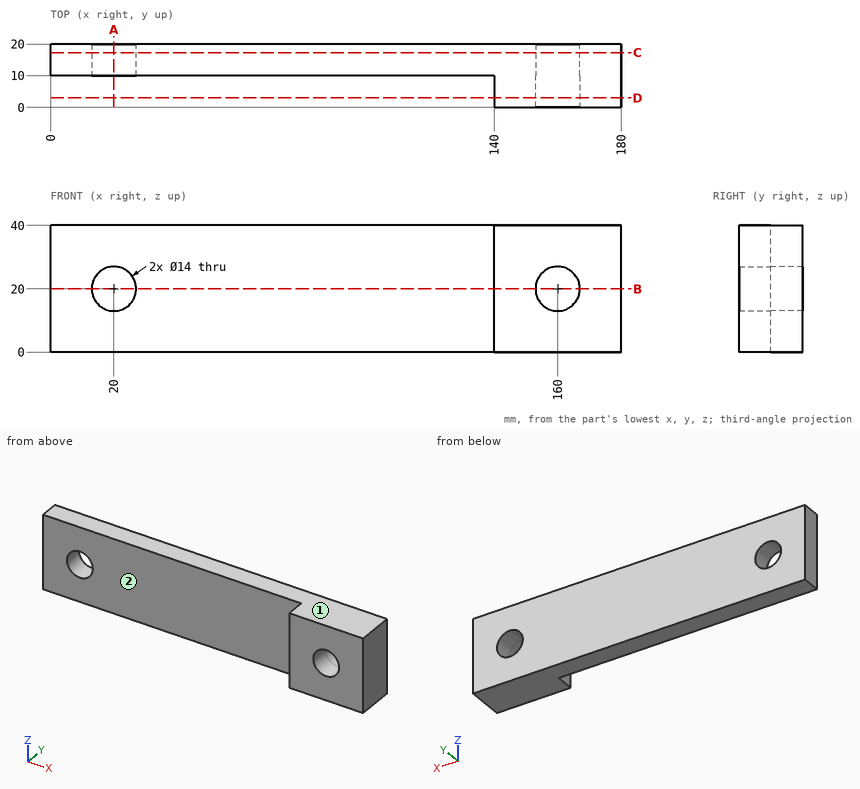
Design review of the part shown in the three views and the two pictorial views. Dimensions are in mm from the part's minimum x, y and z. A direction names the side the tool comes from. Give positions to 0.01 mm unless a question says otherwise; leave off trailing zeros. Write each loop counter-clockwise with the first axis right and the second up, starting at its lowest first coordinate (ties: lowest second). Pieces come first, ordered by that corner, then holes. Notation, with made-up numbers: (-29, 70.25) - (13, 70.25) arc R24 ccw to (13, 90.25) - close; hole circle Ø5 at (14, 33.25). An arc over 180 degrees is marked (long way). Return JSON: item names as keys, results as strings. Group by question number.
(1) Machinability: for the marked faces 1 and 2, which of the approach directions +Z, -Z, +X, -X, +Y, -Y give a long, thin tool a straight path to every point of the face, cutting with its end or side? Answer none if there is none.
(2) We need section D-D, the plane y = 3. Give the boundary of the cut face in (x, z), then the cut area to 3 significant figures.
(3) We need section C-C, the plane y = 17.25. Give the boundary of the cut face in (x, z).
(4) Insertion check: pin 1 (5 mm diameter, centred on y = 4, z = 10.5, fed in from -X); pin 2 (1 mm diameter, centred on x = 47, y = 14, fed in from -Z); pin 3 (20 mm diameter, centred on x = 51.5, z = 20, fed in from -Y); pin 4 (11 mm diameter, centred on x = 160, z = 20, fed in from -Y). Each pin has a flat end and moves straight along its axis. Give the tip position at first contact, or say it passes through.
(5) To check wall thickness, follow probe 1 along X at (y, z) = (16.5, 19.5); probe 2 along Z at (x, y) = (160, 7); probe 3 along X at (y, z) = (10.75, 24). State the ranges of each line that lie inside material, in increasing order.
(6) We need section A-A, the plane x = 20. Give the boundary of the cut face in (y, z), then the cut area to 3 significant figures.
(7) We need section B-B, the plane z = 20. Give the boundary of the cut face in (x, y).
Reported:
{
 "1": {"face 1": "+Z, +X, -X, +Y, -Y", "face 2": "+Z, -Z, -X, -Y"},
 "2": {"outline": "(140, 0) - (180, 0) - (180, 40) - (140, 40) - close; hole circle Ø14 at (160, 20)", "area": "1,450 mm2"},
 "3": {"outline": "(0, 0) - (180, 0) - (180, 40) - (0, 40) - close; hole circle Ø14 at (20, 20); hole circle Ø14 at (160, 20)"},
 "4": {"pin 1": "stops at x = 140", "pin 2": "stops at z = 0", "pin 3": "stops at y = 10", "pin 4": "passes through"},
 "5": {"probe 1": "x = 0 to 13.02, 26.98 to 153.02, 166.98 to 180", "probe 2": "z = 0 to 13, 27 to 40", "probe 3": "x = 0 to 14.26, 25.74 to 154.26, 165.74 to 180"},
 "6": {"outline": "(10, 0) - (20, 0) - (20, 13) - (10, 13) - close; (10, 27) - (20, 27) - (20, 40) - (10, 40) - close", "area": "260 mm2"},
 "7": {"outline": "(0, 10) - (13, 10) - (13, 20) - (0, 20) - close; (27, 10) - (140, 10) - (140, 0) - (153, 0) - (153, 20) - (27, 20) - close; (167, 0) - (180, 0) - (180, 20) - (167, 20) - close"}
}
